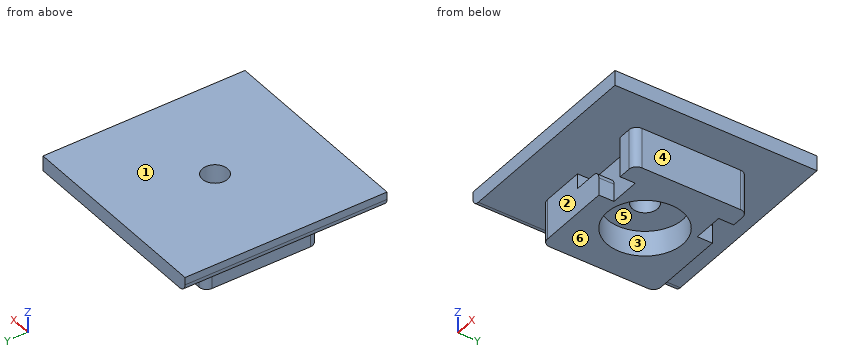
from build123d import *

# Parameters (mm, degrees)
F0_W           = 50.8
F0_H           = 50.8
F1_DEPTH       = 3.81
F3_DEPTH       = 3.81
F5_DEPTH       = 6.35
F6_R           = 1.905
F8_D           = 6.35
F8_CBORE_D     = 19.05
F8_CBORE_DEPTH = 6.35


with BuildPart() as f1:
    # F0 (on Top) → F1 (new body)
    with BuildSketch(Plane.XY):
        Rectangle(F0_W, F0_H)
    extrude(amount=F1_DEPTH)

    # F2 (on face) → F3 (join)
    with BuildSketch(Plane(origin=(0, 0, 0), x_dir=(1, 0, 0), z_dir=(0, 0, -1))):
        Polygon((-3.81, 14.2875), (-16.51, 14.2875), (-16.51, -14.2875), (-3.81, -14.2875), (-3.81, -10.4775), (11.43, -10.4775), (11.43, -14.2875), (16.51, -14.2875), (16.51, 14.2875), (11.43, 14.2875), (11.43, 10.4775), (-3.81, 10.4775), align=None)
    extrude(amount=F3_DEPTH)

    # F4 (on face) → F5 (join)
    with BuildSketch(Plane(origin=(0, 0, -3.81), x_dir=(1, 0, 0), z_dir=(0, 0, -1))):
        Polygon((3.81, 14.2875), (-16.51, 14.2875), (-16.51, -14.2875), (3.81, -14.2875), (3.81, -10.4775), (11.43, -10.4775), (11.43, -14.2875), (16.51, -14.2875), (16.51, 14.2875), (11.43, 14.2875), (11.43, 10.4775), (3.81, 10.4775), align=None)
    extrude(amount=F5_DEPTH)

    # F6
    f6_edges = [f1.edges().sort_by_distance(p)[0] for p in [
        (3.81, -12.3825, -3.81),
        (16.51, -14.2875, -5.08),
        (16.51, 14.2875, -5.08),
        (3.81, 12.3825, -3.81),
        (-16.51, 14.2875, -5.08),
        (-16.51, -14.2875, -5.08),
        (-25.4, 0, 0),
    ]]
    fillet(f6_edges, radius=F6_R)

    # F8 (through all)
    with Locations(Plane(origin=(0, 0, -10.16), x_dir=(1, 0, 0), z_dir=(0, 0, -1))):
        with Locations((0, 0)):
            CounterBoreHole(F8_D / 2, F8_CBORE_D / 2, F8_CBORE_DEPTH)


solid = f1.part
CAD build for the part. Positions are in the model's coordinates, mm. Face numbers are marked on the shaded views. A direction names the side the tool comes from. Round coordinates to 2 decimals unless told otherwise and drop trailing zeros. Write each loop counter-clockwise with the first axis right and the second up, starting at its lowest first coordinate (ties: lowest second). Pieces come first, ordered by that corner, then holes. Notation, with made-up numbers: M -33.5,38.5 L 11.5,38.5 A11 ccw 11.5,54.5 Z; hole C 31,56.5 d6. An arc over 180 degrees is marked long. Use a Markdown table: item, result. Add a question column.
1. Slice it at A-A on x = 0. Give the cut face in (y, z) (1 decimal), then the cut area to 3 significant figures.
2. Slice it at D-D on x = -14. Give the cut face in (y, z), then the cut area to 3 significant figures.
3. Drill centre lines: probe 1 along Y at (x, z) = (0, -0.25) (1 decimal); probe 2 along X at (y, z) = (-11.5, -7.5); probe 3 along Y at (x, z) = (0, -6.5) (1 decimal). Where is each one in solid material? Low to high.
4. Slice it at B-B on y = 0. Give the cut face in (x, z) (3 decimals).
5. Flat gauge pins, fed straight in: P1, Ø1.1, axis at y = -11.5, z = -8, coming from the +X side; P2, Ø22, axis at x = 0, y = 0, coming from the -Z side; P3, Ø1.9, axis at y = 12, z = -4.5, coming from the -X side; P4, Ø1, axis at x = 6, y = 11.5, coming from the -Z side. Where does each tip first touch, or does it go through?
6. Pull direction X, two halves, no side cores. Call the marked faces 4, 5 and 6: released by +X, released by -X, zero draft, split by the parting line, or undercut.
7. 3-axis set-ups, long thin cutter, end or side, ignore diameter. For the marked faces 1, 2 and 3: which of +Z, -Z, +X, -X, +Y, -Y reach the whole face in a straight line?
Reply:
| question | item | result |
|---|---|---|
| 1 | outline | M -25.4,0 L -10.5,0 L -10.5,-3.8 L -14.3,-3.8 L -14.3,-10.2 L -9.5,-10.2 L -9.5,-3.8 L -3.2,-3.8 L -3.2,3.8 L -25.4,3.8 Z; M 3.2,-3.8 L 9.5,-3.8 L 9.5,-10.2 L 14.3,-10.2 L 14.3,-3.8 L 10.5,-3.8 L 10.5,0 L 25.4,0 L 25.4,3.8 L 3.2,3.8 Z |
| 1 | area | 285 mm^2 |
| 2 | outline | M -25.4,0 L -14.29,0 L -14.29,-10.16 L 14.29,-10.16 L 14.29,0 L 25.4,0 L 25.4,3.81 L -25.4,3.81 Z |
| 2 | area | 484 mm^2 |
| 3 | probe 1 | y = -10.5 to -3.2, 3.2 to 10.5 |
| 3 | probe 2 | x = -16.51 to 3.81, 11.43 to 16.51 |
| 3 | probe 3 | y = -14.3 to -9.5, 9.5 to 14.3 |
| 4 | outline | M -25.4,1.905 A1.905 ccw -23.495,0 L -16.51,0 L -16.51,-10.16 L -9.525,-10.16 L -9.525,-3.81 L -3.175,-3.81 L -3.175,3.81 L -25.4,3.81 Z; M 3.175,-3.81 L 9.525,-3.81 L 9.525,-10.16 L 16.51,-10.16 L 16.51,0 L 25.4,0 L 25.4,3.81 L 3.175,3.81 Z |
| 5 | P1 | stops at x = 16.51 |
| 5 | P2 | stops at z = -10.16 |
| 5 | P3 | stops at x = -16.51 |
| 5 | P4 | stops at z = 0 |
| 6 | face 4 | released by +X |
| 6 | face 5 | undercut |
| 6 | face 6 | zero draft |
| 7 | face 1 | +Z, +X, -X, +Y, -Y |
| 7 | face 2 | -Z, +X, -X, -Y |
| 7 | face 3 | -Z |
